```python
from build123d import *

# Parameters (mm, degrees)
SKETCH1_R                         = 4.5
BOSS_EXTRUDE1_DEPTH               = 1.5
BOSS_EXTRUDE2_DEPTH               = 1.5
F_1_0_1_DIAMETER_HOLE1_AT_2_COUNT = 2
F_1_0_1_DIAMETER_HOLE1_AT_2_PITCH = 3.25
F_1_0_1_DIAMETER_HOLE1_AT_3_COUNT = 2
F_1_0_1_DIAMETER_HOLE1_AT_3_PITCH = 6.5
F_1_0_1_DIAMETER_HOLE1_AT_4_COUNT = 2
F_1_0_1_DIAMETER_HOLE1_AT_4_PITCH = 9.75
CIRPATTERN1_COUNT                 = 2
SKETCH6_R                         = 3
CUT_EXTRUDE1_DEPTH                = 0.5
SKETCH7_R                         = 2.5
SKETCH7_R_2                       = 2
EXTRUDE_THIN1_DEPTH               = 0.7
SKETCH8_R                         = 1.25
CUT_EXTRUDE2_DEPTH                = 17.410743432
SKETCH9_R                         = 3.5
BOSS_EXTRUDE3_DEPTH               = 2
CUT_EXTRUDE3_START                = -2.5
SKETCH10_R                        = 3
CUT_EXTRUDE3_DEPTH                = 2.5


with BuildPart() as part:
    # Sketch1 → Boss-Extrude1 (new body)
    with BuildSketch(Plane(origin=(0, 0, 0), x_dir=(1, 0, 0), z_dir=(0, 1, 0))):
        with Locations(Location((0, 0, 0), (0, 0, 270))):
            Circle(SKETCH1_R)
    extrude(amount=BOSS_EXTRUDE1_DEPTH)

    # Sketch2 → Boss-Extrude2 (add)
    with BuildSketch(Plane(origin=(0, 0, 0), x_dir=(1, 0, 0), z_dir=(0, 1, 0))):
        with BuildLine():
            Line((3.5, 2.828427125), (1.729406446, 14.267681426))
            ThreePointArc((1.729406446, 14.267681426), (0, 15.75), (-1.729406446, 14.267681426))
            Line((-1.729406446, 14.267681426), (-3.5, 2.828427125))
            Line((-3.5, 2.828427125), (3.5, 2.828427125))
        make_face()
    boss_extrude2 = extrude(amount=BOSS_EXTRUDE2_DEPTH)

    # Sketch5 → Ø1.0 (1) Diameter Hole1 (revolve, cut)
    with BuildSketch(Plane(origin=(0, 1.5, -14), x_dir=(0, 0, 1), z_dir=(1, 0, 0))):
        Polygon((0, 0), (0, 7.80043031), (0.5, 7.5), (0.5, 0), align=None)
    f_1_0_1_diameter_hole1 = revolve(axis=Axis((0, 7.85, -14), (0, -1, 0)), mode=Mode.SUBTRACT)

    # Ø1.0 (1) Diameter Hole1 at 2: Ø1.0 (1) Diameter Hole1 ×2
    with Locations(*[(0, 0, i * F_1_0_1_DIAMETER_HOLE1_AT_2_PITCH) for i in range(1, F_1_0_1_DIAMETER_HOLE1_AT_2_COUNT)]):
        add(f_1_0_1_diameter_hole1, mode=Mode.SUBTRACT)

    # Ø1.0 (1) Diameter Hole1 at 3: Ø1.0 (1) Diameter Hole1 ×2
    with Locations(*[(0, 0, i * F_1_0_1_DIAMETER_HOLE1_AT_3_PITCH) for i in range(1, F_1_0_1_DIAMETER_HOLE1_AT_3_COUNT)]):
        add(f_1_0_1_diameter_hole1, mode=Mode.SUBTRACT)

    # Ø1.0 (1) Diameter Hole1 at 4: Ø1.0 (1) Diameter Hole1 ×2
    with Locations(*[(0, 0, i * F_1_0_1_DIAMETER_HOLE1_AT_4_PITCH) for i in range(1, F_1_0_1_DIAMETER_HOLE1_AT_4_COUNT)]):
        add(f_1_0_1_diameter_hole1, mode=Mode.SUBTRACT)

    # CirPattern1: Boss-Extrude2, Ø1.0 (1) Diameter Hole1 ×2 about axis
    cirpattern1_axis = Axis((0, 0, 0), (0, 1, 0))
    add([boss_extrude2.rotate(cirpattern1_axis, i * 360 / CIRPATTERN1_COUNT) for i in range(1, CIRPATTERN1_COUNT)])
    add([f_1_0_1_diameter_hole1.rotate(cirpattern1_axis, i * 360 / CIRPATTERN1_COUNT) for i in range(1, CIRPATTERN1_COUNT)], mode=Mode.SUBTRACT)

    # CirPattern1 copy 1 sketch → CirPattern1 copy 1 (revolve, cut)
    with BuildSketch(Plane(origin=(0, 1.5, 10.75), x_dir=(0, 0, -1), z_dir=(-1, 0, 0))):
        Polygon((0, 0), (0, 7.80043031), (0.5, 7.5), (0.5, 0), align=None)
    revolve(axis=Axis((0, 7.85, 10.75), (0, -1, 0)), mode=Mode.SUBTRACT)

    # CirPattern1 copy 2 sketch → CirPattern1 copy 2 (revolve, cut)
    with BuildSketch(Plane(origin=(0, 1.5, 7.5), x_dir=(0, 0, -1), z_dir=(-1, 0, 0))):
        Polygon((0, 0), (0, 7.80043031), (0.5, 7.5), (0.5, 0), align=None)
    revolve(axis=Axis((0, 7.85, 7.5), (0, -1, 0)), mode=Mode.SUBTRACT)

    # CirPattern1 copy 3 sketch → CirPattern1 copy 3 (revolve, cut)
    with BuildSketch(Plane(origin=(0, 1.5, 4.25), x_dir=(0, 0, -1), z_dir=(-1, 0, 0))):
        Polygon((0, 0), (0, 7.80043031), (0.5, 7.5), (0.5, 0), align=None)
    revolve(axis=Axis((0, 7.85, 4.25), (0, -1, 0)), mode=Mode.SUBTRACT)

    # Sketch6 → Cut-Extrude1 (cut)
    with BuildSketch(Plane(origin=(0, 1.5, 0), x_dir=(1, 0, 0), z_dir=(0, 1, 0))):
        with Locations(Location((0, 0, 0), (0, 0, 270))):
            Circle(SKETCH6_R)
    extrude(amount=-CUT_EXTRUDE1_DEPTH, mode=Mode.SUBTRACT)

    # Sketch7 → Extrude-Thin1 (add)
    with BuildSketch(Plane(origin=(0, 1, 0), x_dir=(1, 0, 0), z_dir=(0, 1, 0))):
        Circle(SKETCH7_R)
        Circle(SKETCH7_R_2, mode=Mode.SUBTRACT)
    extrude(amount=EXTRUDE_THIN1_DEPTH)

    # Sketch8 → Cut-Extrude2 (cut, through all)
    with BuildSketch(Plane(origin=(0, 1, 0), x_dir=(1, 0, 0), z_dir=(0, 1, 0))):
        with Locations(Location((0, 0, 0), (0, 0, 270))):
            Circle(SKETCH8_R)
    extrude(amount=-CUT_EXTRUDE2_DEPTH, mode=Mode.SUBTRACT)

    # Sketch9 → Boss-Extrude3 (add)
    with BuildSketch(Plane.XZ):
        with Locations(Location((0, 0, 0), (0, 0, 90))):
            Circle(SKETCH9_R)
    extrude(amount=BOSS_EXTRUDE3_DEPTH)

    # Sketch10 → Cut-Extrude3 (cut)
    with BuildSketch(Plane.XZ.offset(2).offset(CUT_EXTRUDE3_START)):
        with Locations(Location((0, 0, 0), (0, 0, 90))):
            Circle(SKETCH10_R)
    extrude(amount=CUT_EXTRUDE3_DEPTH, mode=Mode.SUBTRACT)


solid = part.part
```
Read the model definition and answer for the solid it produces. Units are mm, in the model's axes. A direction names the side the tool comes from. Round coordinates to 2 decimals unless told otherwise and drop trailing zeros. Loops run counter-clockwise (first coordinate to the right, second up) from the corner with the lowest first, then second, coordinate; pieces in that order, holes last. Notation, with made-up numbers: (16.5, 23) -> (50.5, 23) arc R30 cw to (50.5, 58) -> close; hole circle Ø1 at (-26.5, 41.5). An arc over 180 degrees is marked (long way). One line per item, written item: value.
1) The mould has two halves that part along Z. Classify faces 4 (the face through (2.6, 0.74, 8.63)), 5 (the face through (2.627, 0.74, -8.468)), 6 (the face through (2, 1, -2)): pulls with the +Z half, pulls with the -Z half, needs draft (parallel to the pull), parting line crosses it, or undercut.
Answer list:
face 4: pulls with the +Z half
face 5: pulls with the -Z half
face 6: undercut
2) A cutting plane is placed at C-C (z = 7.5). Determine the outline of the cut face in (x, y).
Answer list:
outline: (-2.78, 0) -> (-0.5, 0) -> (-0.5, 1.5) -> (-2.78, 1.5) -> close; (0.5, 0) -> (2.78, 0) -> (2.78, 1.5) -> (0.5, 1.5) -> close
3) A cutting plane is placed at D-D (z = 13). Determine the outline of the cut face in (x, y).
Answer list:
outline: (-1.93, 0) -> (1.93, 0) -> (1.93, 1.5) -> (-1.93, 1.5) -> close
4) Flat-ended cylindrical pins translate along their axes: P1, Ø3.5, axis at x = 0, z = 0, coming from the +Y side; P2, Ø5, axis at x = 0, z = 0, coming from the -Y side; P3, Ø1.2, axis at x = 0, z = 0, coming from the +Y side. Find the tip coordinate at first contact, or state that the pin passes through.
Answer list:
P1: stops at y = 1
P2: stops at y = 0.5
P3: passes through
5) For faces 1 (the face through (-1, 1.7, -2)), 2 (the face through (-0.54, 1.35, 2.44)), 3 (the face through (-0.9, -0.73, 2.86)), determine the directions among +Z, -Z, +X, -X, +Y, -Y from which every point of the face is accessible in a straight line to the end or side of a thin tool.
Answer list:
face 1: +Z, -Z, +X, -X, +Y
face 2: +Y
face 3: -Y
6) Consider L1, parallel to Y at x = 1.5, z = -1; L2, parallel to X at y = 0.9, z = 0; L3, parallel to Y at x = 1.5, z = 3.5. Determine where each line is inside the solid, lowest interval first. Write a range as [from, to].
Answer list:
L1: y = [0.5, 1]
L2: x = [-4.5, -1.25], [1.25, 4.5]
L3: y = [0, 1.5]
7) A cutting plane is placed at A-A (z = 0). Determine the outline of the cut face in (x, y), and give its area (3 significant figures).
Answer list:
outline: (-4.5, 0) -> (-3.5, 0) -> (-3.5, -2) -> (-3, -2) -> (-3, 0.5) -> (-1.25, 0.5) -> (-1.25, 1) -> (-2, 1) -> (-2, 1.7) -> (-2.5, 1.7) -> (-2.5, 1) -> (-3, 1) -> (-3, 1.5) -> (-4.5, 1.5) -> close; (1.25, 0.5) -> (3, 0.5) -> (3, -2) -> (3.5, -2) -> (3.5, 0) -> (4.5, 0) -> (4.5, 1.5) -> (3, 1.5) -> (3, 1) -> (2.5, 1) -> (2.5, 1.7) -> (2, 1.7) -> (2, 1) -> (1.25, 1) -> close
area: 8.95 mm²
8) A cutting plane is placed at B-B (y = -0.6). Determine the outline of the cut face in (x, z), and give its area (3 significant figures).
Answer list:
outline: circle Ø7 at (0, 0); hole circle Ø6 at (0, 0)
area: 10.2 mm²
